Input: part model. Units: mm. Frame: model coordinates. A direction names the side the tool comes from. Coordinates: 2 decimals unless noted, no trailing zeros. Order: outer loops, then holes, each group sorted by start corner. A loop starts at its lowest first (then second) coordinate and runs counter-clockwise, first axis right, second up. Notation, with made-up numbers: (83, -19) -> (125, -19) arc R27 cw to (125, 18) -> close; hole circle Ø9 at (8.5, 63.5). An arc over 180 degrees is marked (long way). Use CSV: the item, a comma, the result in double quotes. Start each with the question number.
```python
from build123d import *

# Parameters (mm, degrees)
F1_DEPTH = 6.35
F2_DEPTH = 50.8


with BuildPart() as f1:
    # F0 (on Top) → F1 (new body)
    with BuildSketch(Plane.XY):
        Polygon((3.252794, 21.851061), (3.252794, 22.285081), (3.252794, 24.165833), (1.082697, 24.165833), (1.082697, 26.480602), (-1.232074, 26.480602), (-1.232074, 28.795373), (-3.402171, 28.795373), (-6.440307, 28.795373), (-9.189097, 28.795373), (-9.189097, 26.480602), (-11.64854, 26.480602), (-11.64854, 24.165833), (-13.818637, 24.165833), (-13.818637, 22.285081), (-16.133409, 22.285081), (-16.133409, 18.812926), (-14.976023, 18.812926), (-14.976023, 15.630117), (-13.529291, 15.630117), (-13.529291, 11.000575), (-11.64854, 11.000575), (-11.64854, 7.0944), (-7.742365, 7.0944), (-7.742365, 4.345611), (-3.402171, 4.345611), (-3.402171, 2.03084), (0, 2.03084), (0, 0), (1.082697, 0), (1.082697, -2.309354), (4.265506, -2.309354), (4.265506, 0), (6.580276, 0), (6.580276, 2.03084), (9.329067, 2.03084), (9.329067, 4.200937), (12.511875, 4.200937), (12.511875, 7.673093), (15.550012, 7.673093), (15.550012, 9.553844), (18.443475, 9.553844), (18.443475, 13.894038), (19.890206, 13.894038), (19.890206, 18.668253), (21.192264, 18.668253), (21.192264, 23.442466), (19.022167, 23.442466), (19.022167, 25.178544), (17.430764, 25.178544), (17.430764, 27.637988), (15.839359, 27.637988), (15.839359, 29.374065), (9.329067, 29.374065), (9.329067, 26.914621), (7.737662, 26.914621), (7.737662, 24.310505), (5.856911, 24.310505), (5.856911, 21.851061), align=None)
    extrude(amount=F1_DEPTH)

    # F0 (on Top) → F2 (join)
    with BuildSketch(Plane.XY):
        Polygon((0, 28.223222), (0, 30.817736), (-10.882908, 30.817736), (-10.882908, 27.677011), (-13.887079, 27.677011), (-13.818637, 26.480602), (-15.930331, 26.359802), (-15.804824, 24.165833), (-18.256783, 24.165833), (-18.256783, 17.435515), (-16.071932, 17.435515), (-16.071932, 13.06581), (-14.979505, 13.06581), (-14.979505, 9.515426), (-13.818637, 9.515426), (-13.818637, 5.828488), (-9.517374, 5.828488), (-9.517374, 2.414656), (-5.693883, 2.414656), (-5.693883, 0), (-1.870391, 0), (-1.870391, -3.866795), (0, -3.866795), (0, -6.188201), (6.186252, -6.188201), (6.186252, -2.309354), (8.917317, -2.228155), (8.85107, 0), (11.64057, 0.082936), (11.571244, 2.414656), (14.78221, 2.510123), (14.687699, 5.688919), (18.212094, 5.793705), (18.142457, 8.135915), (20.526713, 8.206803), (20.387793, 11.973385), (22.019175, 12.033554), (22.162985, 16.616195), (24.341406, 16.547833), (24.341406, 25.082497), (21.616772, 25.082497), (21.616772, 26.448032), (19.568473, 26.448032), (19.568473, 29.31565), (17.929833, 29.31565), (17.929833, 31.363949), (7.688338, 31.363949), (7.688338, 28.144343), (5.913145, 28.144343), (5.913145, 26.914621), (3.455187, 26.914621), (3.455187, 28.223222), align=None)
        Polygon((3.252794, 24.165833), (3.252794, 22.285081), (3.252794, 21.851061), (5.856911, 21.851061), (5.856911, 24.310505), (7.737662, 24.310505), (7.737662, 26.914621), (9.329067, 26.914621), (9.329067, 29.374065), (15.839359, 29.374065), (15.839359, 27.637988), (17.430764, 27.637988), (17.430764, 25.178544), (19.022167, 25.178544), (19.022167, 23.442466), (21.192264, 23.442466), (21.192264, 18.668253), (19.890206, 18.668253), (19.890206, 13.894038), (18.443475, 13.894038), (18.443475, 9.553844), (15.550012, 9.553844), (15.550012, 7.673093), (12.511875, 7.673093), (12.511875, 4.200937), (9.329067, 4.200937), (9.329067, 2.03084), (6.580276, 2.03084), (6.580276, 0), (4.265506, 0), (4.265506, -2.309354), (1.082697, -2.309354), (1.082697, 0), (0, 0), (0, 2.03084), (-3.402171, 2.03084), (-3.402171, 4.345611), (-7.742365, 4.345611), (-7.742365, 7.0944), (-11.64854, 7.0944), (-11.64854, 11.000575), (-13.529291, 11.000575), (-13.529291, 15.630117), (-14.976023, 15.630117), (-14.976023, 18.812926), (-16.133409, 18.812926), (-16.133409, 22.285081), (-13.818637, 22.285081), (-13.818637, 24.165833), (-11.64854, 24.165833), (-11.64854, 26.480602), (-9.189097, 26.480602), (-9.189097, 28.795373), (-6.440307, 28.795373), (-3.402171, 28.795373), (-1.232074, 28.795373), (-1.232074, 26.480602), (1.082697, 26.480602), (1.082697, 24.165833), align=None, mode=Mode.SUBTRACT)
    extrude(amount=F2_DEPTH)


solid = f1.part
```
1. Contact query for flat-ended pins moving along their axis: P1, Ø0.7, axis at y = 26, z = 13, coming from the +X side; P2, Ø2.5, axis at y = 25.5, z = 32.5, coming from the -X side; P3, Ø1, axis at y = 0.5, z = 25.5, coming from the +X side; P4, Ø1.4, axis at y = 24.5, z = 30, coming from the -X side. Output: stop coordinate, or through.
2. Pull-direction query (Y, two-part tool) for faces 1 (the face through (23, 25.082, 25)), 2 (the face through (5.913, 27.5, 25)), 3 (the face through (3.253, 23, 28)); classes: released by +Y, released by -Y, zero draft, split by the parting line, or undercut.
3. Material intervals for line 1 along Y through (x, z) = (-1, 32); line 2 along X through (y, z) = (8, 48); line 3 along Y through (x, z) = (-6.5, 37.5), sorted ascending.
4. Section A-A on x = -5. Return loops of the section in (y, z), then the cut area to 3 significant figures.
5. Section B-B on y = 20. Return loops of the section in (x, z), then the cut area to 3 significant figures.
6. Access query for faces 4 (the face through (21, 26.448, 25)), 5 (the face through (5, 0, 28)), 6 (the face through (7, 28.144, 25)), 7 (the face through (3, -6.188, 25)), 8 (the face through (-12, 27.677, 25)). Directions: +Z, -Z, +X, -X, +Y, -Y. A direction counts if a zero-diameter tool reaches every point of the face in a straight line with its end or side. Return the directions, or none.
Values follow:
1,P1,"stops at x = 21.62"
1,P2,"stops at x = -15.93"
1,P3,"stops at x = 11.64"
1,P4,"stops at x = -18.26"
2,face 1,"released by +Y"
2,face 2,"zero draft"
2,face 3,"undercut"
3,line 1,"y = -3.87 to 2.03, 26.48 to 30.82"
3,line 2,"x = -13.82 to -11.65, 15.55 to 18.15"
3,line 3,"y = 2.41 to 4.35, 28.8 to 30.82"
4,outline,"(0, 0) -> (30.82, 0) -> (30.82, 50.8) -> (28.8, 50.8) -> (28.8, 6.35) -> (4.35, 6.35) -> (4.35, 50.8) -> (0, 50.8) -> close"
4,area,"479 mm2"
5,outline,"(-18.26, 0) -> (24.34, 0) -> (24.34, 50.8) -> (21.19, 50.8) -> (21.19, 6.35) -> (-16.13, 6.35) -> (-16.13, 50.8) -> (-18.26, 50.8) -> close"
5,area,"505 mm2"
6,face 4,"+Z, -Z, +X, +Y"
6,face 5,"+Z"
6,face 6,"+Z, -Z, +Y"
6,face 7,"+Z, -Z, +X, -X, -Y"
6,face 8,"+Z, -Z, -X, +Y"
